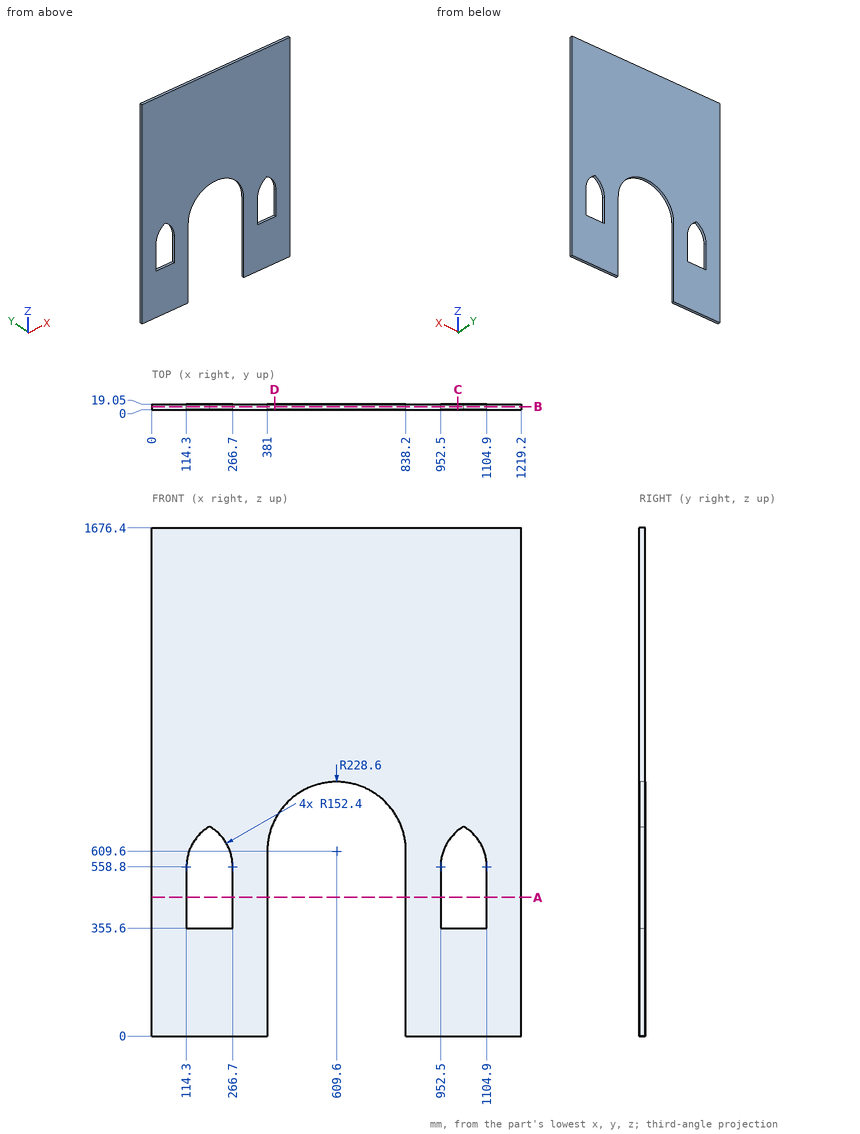
Could you check a few things on this drawing? It's one solid part, dimensions in mm from its lowest x, y, z. Give positions to 0.01 mm unless a question says otherwise; leave off trailing zeros. Order: outer loops, then holes, each group sorted by start corner. A loop starts at its lowest first (then second) coordinate and runs counter-clockwise, first axis right, second up. Notation, with made-up numbers: (-36, 3.5) - (3, 3.5) arc R23 cw to (3, 38.5) - close; hole circle Ø4 at (62.25, 32.5). An arc over 180 degrees is marked (long way). Return JSON: item names as keys, results as strings. Group by question number.
Q1. Suppose I cut it at A-A, the plane z = 457. Please give me the cut outline in (x, y).
Q2. Suppose I cut it at C-C, the plane x = 1009.5. Please give me the cut outline in (y, z).
Q3. Please list where these lines run through material, in increasing order: line 1 along X through (y, z) = (14.5, 526.5); line 2 along X through (y, z) = (1.5, 269.5); line 3 along Z through (x, y) = (245, 9.25). Write a range as [from, to].
Q4. Suppose I cut it at B-B, the plane y = 10.75. Please give me the cut outline in (x, z).
Q5. Suppose I cut it at D-D, the plane x = 405. Please give me the cut outline in (y, z).
Resolved:
{
 "1": {"outline": "(0, 0) - (114.3, 0) - (114.3, 19.05) - (0, 19.05) - close; (266.7, 0) - (381, 0) - (381, 19.05) - (266.7, 19.05) - close; (838.2, 0) - (952.5, 0) - (952.5, 19.05) - (838.2, 19.05) - close; (1104.9, 0) - (1219.2, 0) - (1219.2, 19.05) - (1104.9, 19.05) - close"},
 "2": {"outline": "(0, 0) - (19.05, 0) - (19.05, 355.6) - (0, 355.6) - close; (0, 677.65) - (19.05, 677.65) - (19.05, 1676.4) - (0, 1676.4) - close"},
 "3": {"line 1": "x = [0, 114.3], [266.7, 381], [838.2, 952.5], [1104.9, 1219.2]", "line 2": "x = [0, 381], [838.2, 1219.2]", "line 3": "z = [0, 355.6], [637.18, 1676.4]"},
 "4": {"outline": "(0, 0) - (381, 0) - (381, 609.6) arc R228.6 cw to (838.2, 609.6) - (838.2, 0) - (1219.2, 0) - (1219.2, 1676.4) - (0, 1676.4) - close; hole (114.3, 355.6) - (266.7, 355.6) - (266.7, 558.8) arc R152.4 ccw to (190.5, 690.78) arc R152.4 ccw to (114.3, 558.8) - close; hole (952.5, 355.6) - (1104.9, 355.6) - (1104.9, 558.8) arc R152.4 ccw to (1028.7, 690.78) arc R152.4 ccw to (952.5, 558.8) - close"},
 "5": {"outline": "(0, 711.56) - (19.05, 711.56) - (19.05, 1676.4) - (0, 1676.4) - close"}
}
